```python
from build123d import *

# Parameters (mm, degrees)
F0_W     = 43.1823767722
F0_H     = 24.0973075852
F4_R     = 5.7616257058
F5_DEPTH = 30


# Not quite as in the source:
# - the arcs of a loft's sections are written as splines that run evenly, so that the points pair up as in the source's solid


with BuildPart() as f3:
    # F2 (on offset) → F3 section 0
    with BuildSketch(Plane.XY.offset(30)):
        with BuildLine():
            add(Edge.make_bspline(
                [(-14.3525502898, -6.4258121346), (-13.7994999926, -7.3651843545), (-13.1539455701, -8.2500639934), (-11.7025735307, -9.8769193643), (-10.8967918018, -10.618854869), (-9.1559237309, -11.9313020315), (-8.2208804354, -12.5017812365), (-6.2574169169, -13.4493835823), (-5.2290452443, -13.8264832918), (-3.1184410799, -14.3728249941), (-2.036260777, -14.5420534776), (0.1403746989, -14.6661389313), (1.2347760501, -14.6209928331), (3.3937959567, -14.3180535037), (4.4583611261, -14.0602677631), (6.5167955393, -13.3419454391), (7.5106138842, -12.8814266176), (8.449986104, -12.3283763204)],
                knots=[0, 0, 0, 0, 0.125, 0.125, 0.25, 0.25, 0.375, 0.375, 0.5, 0.5, 0.625, 0.625, 0.75, 0.75, 0.875, 0.875, 1, 1, 1, 1], degree=3))
            add(Edge.make_bspline(
                [(8.449986104, -12.3283763204), (9.3893583239, -11.7753260232), (10.2742379628, -11.1297716007), (11.9010933337, -9.6783995613), (12.6430288384, -8.8726178324), (13.9554760009, -7.1317497615), (14.5259552059, -6.196706466), (15.4735575517, -4.2332429475), (15.8506572612, -3.2048712749), (16.3969989635, -1.0942671105), (16.566227447, -0.0120868075), (16.6903129007, 2.1645486683), (16.6451668025, 3.2589500195), (16.3422274731, 5.4179699262), (16.0844417325, 6.4825350955), (15.3661194086, 8.5409695087), (14.905600587, 9.5347878536), (14.3525502898, 10.4741600735)],
                knots=[0, 0, 0, 0, 0.125, 0.125, 0.25, 0.25, 0.375, 0.375, 0.5, 0.5, 0.625, 0.625, 0.75, 0.75, 0.875, 0.875, 1, 1, 1, 1], degree=3))
            add(Edge.make_bspline(
                [(14.3525502898, 10.4741600735), (13.7994999926, 11.4135322933), (13.1539455701, 12.2984119322), (11.7025735307, 13.9252673031), (10.8967918018, 14.6672028078), (9.1559237309, 15.9796499703), (8.2208804354, 16.5501291753), (6.2574169169, 17.4977315211), (5.2290452443, 17.8748312306), (3.1184410799, 18.4211729329), (2.036260777, 18.5904014164), (-0.1403746989, 18.7144868701), (-1.2347760501, 18.6693407719), (-3.3937959567, 18.3664014425), (-4.4583611261, 18.108615702), (-6.5167955393, 17.390293378), (-7.5106138842, 16.9297745564), (-8.449986104, 16.3767242592)],
                knots=[0, 0, 0, 0, 0.125, 0.125, 0.25, 0.25, 0.375, 0.375, 0.5, 0.5, 0.625, 0.625, 0.75, 0.75, 0.875, 0.875, 1, 1, 1, 1], degree=3))
            add(Edge.make_bspline(
                [(-8.449986104, 16.3767242592), (-9.3893583239, 15.823673962), (-10.2742379628, 15.1781195395), (-11.9010933337, 13.7267475001), (-12.6430288384, 12.9209657712), (-13.9554760009, 11.1800977003), (-14.5259552059, 10.2450544049), (-15.4735575517, 8.2815908863), (-15.8506572612, 7.2532192137), (-16.3969989635, 5.1426150493), (-16.566227447, 4.0604347464), (-16.6903129007, 1.8837992705), (-16.6451668025, 0.7893979193), (-16.3422274731, -1.3696219873), (-16.0844417325, -2.4341871567), (-15.3661194086, -4.4926215699), (-14.905600587, -5.4864399148), (-14.3525502898, -6.4258121346)],
                knots=[0, 0, 0, 0, 0.125, 0.125, 0.25, 0.25, 0.375, 0.375, 0.5, 0.5, 0.625, 0.625, 0.75, 0.75, 0.875, 0.875, 1, 1, 1, 1], degree=3))
        make_face()
    # F0 (on Top) → F3 section 1
    with BuildSketch(Plane.XY):
        with Locations((-0.6747245789, 0.963892322)):
            Rectangle(F0_W, F0_H)
    loft(ruled=True)

    # F4 (on face) → F5 (cut)
    with BuildSketch(Plane.XY.offset(30)):
        Circle(F4_R)
    extrude(amount=-F5_DEPTH, mode=Mode.SUBTRACT)


solid = f3.part
```
Can you work these out from the model? Positions are in its coordinate system, mm. Coordinates: 2 decimals unless noted, no trailing zeros. Put each result on its own line as item: value. Start each with the question number.
Q1. If I drill on line 1 (X direction, y = 4, z = 3); line 2 (Y direction, x = -1.5, z = 21.5); line 3 (Y direction, x = 0, z = 7), over which ranges is the centre line in solid material (lowest first)? Write a range as [from, to].
Q2. Thinking about a two-plate mould opening in X: for faces 1 (the face through (2, 7, 0)), 2 (the face through (-5.756, 0.253, 15.21)), which applies, pulls with the +X half, pulls with the -X half, needs draft (parallel to the pull), parting line crosses it, or undercut?
Q3. I'm going to push flat-ended pins straight in: P1, Ø5, axis at y = 12, z = 11.5, coming from the -X side; P2, Ø3, axis at x = -5.5, z = 5.5, coming from the -Y side; P3, Ø2, axis at x = -0.5, z = 8.5, coming from the -Y side; P4, Ø3, axis at x = 12, y = -9.5, coming from the -Z side. Where does each tip first touch, or does it pass through?
Taken from the geometry:
1. line 1: x = [-21.56, -4.15], [4.15, 20.49]
1. line 2: y = [-13.46, -5.56], [5.56, 17.07]
1. line 3: y = [-11.84, -5.76], [5.76, 14.23]
2. face 1: needs draft
2. face 2: undercut
3. P1: stops at x = -18.97
3. P2: stops at y = -11.61
3. P3: stops at y = -12.11
3. P4: stops at z = 0
